Geometry: final body of the model. Coordinates: model frame, mm. Round coordinates to 2 decimals unless told otherwise and drop trailing zeros. Loops run counter-clockwise (first coordinate to the right, second up) from the corner with the lowest first, then second, coordinate; pieces in that order, holes last. Notation, with made-up numbers: M -6.75,-5.5 L 51.25,-5.5 A11 ccw 51.25,7.5 Z; hole C -17,25 d1. An arc over 180 degrees is marked long. Return JSON: item names as keys, results as strings.
Autodesk Inventor part; units mm, degrees
ref_plane "YZ Plane" through (0, 0, 0) normal (1, 0, 0) x (0, 1, 0)
ref_plane "XZ Plane" through (0, 0, 0) normal (0, 1, 0) x (-1, 0, 0)
ref_plane "XY Plane" through (0, 0, 0) normal (0, 0, 1) x (1, 0, 0)
sketch "Sketch1" plane through (0, 0, 0) normal (0, 0, 1) x (1, 0, 0)
  line L0 (0, 0) -> (-6.35, 6.5628)
  line L1 (-6.35, 6.5628) -> (-103.0723, 4.8744)
  line L2 (0, 0) -> (-6.5628, -6.35)
  line L3 (-6.5628, -6.35) -> (-103.1769, -1.4756)
  arc A0 (-103.0723, 4.8744) -> (-103.1769, -1.4756) centre (0, 0) ccw
  dimension "d0" = 103.1875
  dimension "d1" = 6.35
  dimension "d2" = 6.35
  dimension "d3" = 133.056
  dimension "d4" = 133.056
extrude "Extrusion1" add sketch "Sketch1" along normal blind 6.35
fillet "Fillet1" radius 3.81 2 edges at (-54.8699, -3.9128, 6.35) (-54.7112, 5.7186, 6.35)
properties part number "Lift_Support"
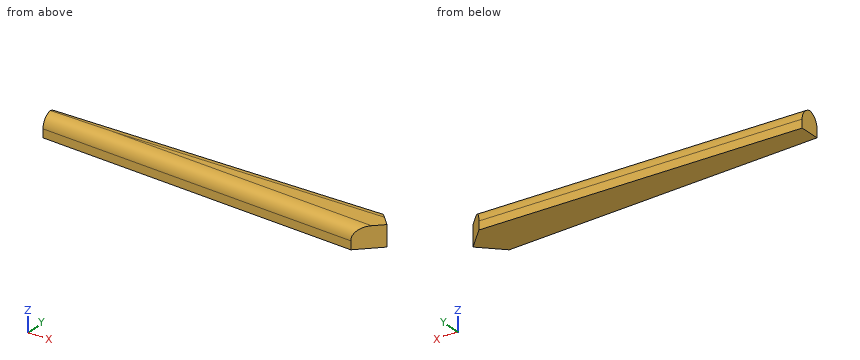
Q1. Material intervals for L1, parallel to X at y = 0, z = 0.5; L2, parallel to Z at x = -56.5, y = 2.25; L3, parallel to Y at x = -19.5, z = 3.5, sorted ascending.
Determined:
{"L1": "x = -103.19 to 0", "L2": "z = 0 to 6.33", "L3": "y = -5.57 to 6.21"}
Q2. Section query B-B (z = 5.25). Output: boundary loops of the cut face in (x, y).
Determined:
{"outline": "M -103.19,-0.34 L -5.45,-5.27 L 0,0 L -5.27,5.45 L -103.12,3.74 A103.14 ccw Z"}
Q3. Section query A-A (z = 1). Output: boundary loops of the cut face in (x, y).
Determined:
{"outline": "M -103.18,-1.48 L -6.56,-6.35 L 0,0 L -6.35,6.56 L -103.07,4.87 A103.14 ccw Z"}
